Verification items for the finished model (mm, model axes). A direction names the side the tool comes from. Coordinates: 2 decimals unless noted, no trailing zeros. Order: outer loops, then holes, each group sorted by start corner. A loop starts at its lowest first (then second) coordinate and runs counter-clockwise, first axis right, second up.
Q1. Depth check by flat-ended pin: P1, Ø3, axis at y = -204, z = 6.5, coming from the -X side; P2, Ø4, axis at x = 153, y = -250, coming from the -Z side; P3, Ø1.5, axis at x = 183.5, z = 12.5, coming from the +Y side; P4, Ø5, axis at x = 90, z = 8.5, coming from the -Y side. Enter the tip coordinate at first touch or a pass-through.
Q2. Cross-section at C-C, the plane y = -128. Record the boundary of the cut face in (x, z).
Q3. Cross-section at B-B, the plane x = 195. Record the boundary of the cut face in (y, z), and give its area (3 significant figures).
Q4. Draft check along Z on faces 3 (the flat face through (203, -213, 25.4)), 4 (the flat face through (212, -212, 1.588)), 5 (the cylindrical face through (208.596, -204.476, 12.522)). Enter one of: pulls with the +Z half, pulls with the -Z half, needs draft (parallel to the pull), parting line crosses it, or undercut.
Q5. Cross-section at A-A, the plane z = 13. Record the boundary of the cut face in (x, y).
Q6. Set-up check for faces 1 (the flat face through (304, -25.4, 1)), 2 (the cylindrical face through (226.34, -220.39, 12.54)): record each of +Z, -Z, +X, -X, +Y, -Y from which the full face is reachable in a straight line by a thin tool's end or side.
Q7. Thickness scan on line 1 (Z direction, x = 296, y = -106); line 2 (Y direction, x = 248, z = 20.25); line 3 (Y direction, x = 110, z = 10). Record the ranges inside material, lowest first.
Autodesk Inventor part; units mm, degrees
ref_plane "YZ Plane" through (0, 0, 0) normal (1, 0, 0) x (0, 1, 0)
ref_plane "XZ Plane" through (0, 0, 0) normal (0, 1, 0) x (-1, 0, 0)
ref_plane "XY Plane" through (0, 0, 0) normal (0, 0, 1) x (1, 0, 0)
sketch "Sketch1" plane through (0, 0, 0) normal (0, 0, 1) x (1, 0, 0)
  arc A0 (25.5164, -290.9834) -> (290.9936, -25.4) centre (0, 0) ccw
  arc A1 (27.7352, -316.2863) -> (316.4824, -25.4) centre (0, 0) ccw
  line L0 (25.5164, -290.9834) -> (27.7352, -316.2863)
  line L1 (290.9936, -25.4) -> (316.4824, -25.4)
  line L2 (0, 0) -> (25.5164, -290.9834) construction
  line L3 (0, -292.1) -> (0, 0) construction
  line L4 (290.9936, -25.4) -> (0, 0) construction
  line L5 (290.9936, 0) -> (316.4824, 0) construction
  line L6 (316.4824, 0) -> (316.4824, -25.4) construction
  line L7 (316.4824, -25.4) -> (290.9936, -25.4) construction
  line L8 (290.9936, -25.4) -> (290.9936, 0) construction
  line L9 (0, 0) -> (359.7285, 0) construction
  dimension "d0" = 292.1
  dimension "d1" = 25.4
  dimension "d9" = 25.4
  dimension "d10" = 80
extrude "Extrusion1" add sketch "Sketch1" along normal blind 25.4
shell "Shell1" thickness 1.5875 removed faces 2 at (299.4898, -25.4, 8.4667) at (26.9956, -307.852, 16.9333)
properties part number "Shooter_Frame_RearGuide" material "Aluminum-6061"
Check values:
1. P1: stops at x = 207.59
1. P2: stops at z = 0
1. P3: stops at y = -226.66
1. P4: stops at y = -305.2
2. outline: (262.56, 0) - (290.56, 0) - (290.56, 25.4) - (262.56, 25.4) - close; hole (264.33, 1.59) - (288.82, 1.59) - (288.82, 23.81) - (264.33, 23.81) - close
3. outline: (-250.56, 0) - (-217.48, 0) - (-217.48, 25.4) - (-250.56, 25.4) - close; hole (-248.55, 1.59) - (-219.61, 1.59) - (-219.61, 23.81) - (-248.55, 23.81) - close
3. area: 197 mm2
4. face 3: pulls with the +Z half
4. face 4: undercut
4. face 5: needs draft
5. outline: (25.52, -290.98) - (25.66, -292.56) arc R293.69 ccw to (292.59, -25.4) - (290.99, -25.4) arc R292.1 cw to start; (27.6, -314.7) - (27.74, -316.29) arc R317.5 ccw to (316.48, -25.4) - (314.89, -25.4) arc R315.91 cw to start
6. face 1: +Z, -Z, +X, -X, +Y
6. face 2: none
7. line 1: z = 0 to 1.59, 23.81 to 25.4
7. line 2: y = -198.25 to -195.7, -157.32 to -154.33
7. line 3: y = -297.84 to -296.14, -272.31 to -270.6
